Model file for the job. Use its own axes, mm. A direction names the side the tool comes from. Round coordinates to 2 decimals unless told otherwise and drop trailing zeros. Write each loop counter-clockwise with the first axis right and the second up, starting at its lowest first coordinate (ties: lowest second). Pieces come first, ordered by that corner, then holes.
```python
from build123d import *

# Parameters (mm, degrees)
F0_R     = 6.35
F1_DEPTH = 7.62
F2_R     = 3.048
F3_DEPTH = 19.05
F4_R     = 3.048
F5_DEPTH = 19.05


with BuildPart() as f1:
    # F0 (on Front) → F1 (new body)
    with BuildSketch(Plane.XZ):
        Circle(F0_R)
    extrude(amount=F1_DEPTH)

    # F2 (on face) → F3 (join)
    with BuildSketch(Plane(origin=(0, 0, 0), x_dir=(-1, 0, 0), z_dir=(0, 1, 0))):
        Circle(F2_R)
    extrude(amount=F3_DEPTH)

    # F4 (on face) → F5 (join)
    with BuildSketch(Plane.XZ.offset(7.62)):
        Circle(F4_R)
    extrude(amount=F5_DEPTH)


solid = f1.part
```
1) Cut at D-D on z = -3.75. List the corners of the cut face in (x, y), and give its area (3 significant figures).
2) Cut at B-B on x = 0. List the corners of the cut face in (y, z), and give its area (3 significant figures).
3) Cut at A-A on z = 0. List the corners of the cut face in (x, y), and give its area (3 significant figures).
4) Which spindle directions (+Z, -Z, +X, -X, +Y, -Y) get a long thin tool onto all of the face, cutting with end or side? Do faces 3 (the face through (0, -26.67, 0)), 4 (the face through (-0.4, -17.01, 3.02)), 5 (the face through (3, 0, 2)). Say none if no direction does.
5) Flat gauge pins, fed straight in: pin 1 Ø6 at (y, z) = (14.5, 3.5) entering from -X; pin 2 Ø5 at (x, y) = (5, -15) entering from +Z; pin 3 Ø1.5 at (y, z) = (-5.5, -3.5) entering from +X. Where does each tip first touch, or does it go through?
6) Cut at C-C on y = -15.5. List the corners of the cut face in (x, z), and give its area (3 significant figures).
7) Pull direction X, two halves, no side cores. Call faces 1 (the face through (-1.38, -3.76, -6.2)), 2 (the face through (0, 19.05, 0)): released by +X, released by -X, zero draft, split by the parting line, or undercut.
8) Wall check: probe 1 along Y at (x, z) = (-2.75, 5); probe 2 along Z at (x, y) = (-0.25, -20); probe 3 along X at (y, z) = (-1, -5.25). Give the ranges that are in metal, low to high.
Result sheet:
1. outline: (-5.12, -7.62) - (5.12, -7.62) - (5.12, 0) - (-5.12, 0) - close
1. area: 78.1 mm2
2. outline: (-26.67, -3.05) - (-7.62, -3.05) - (-7.62, -6.35) - (0, -6.35) - (0, -3.05) - (19.05, -3.05) - (19.05, 3.05) - (0, 3.05) - (0, 6.35) - (-7.62, 6.35) - (-7.62, 3.05) - (-26.67, 3.05) - close
2. area: 329 mm2
3. outline: (-6.35, -7.62) - (-3.05, -7.62) - (-3.05, -26.67) - (3.05, -26.67) - (3.05, -7.62) - (6.35, -7.62) - (6.35, 0) - (3.05, 0) - (3.05, 19.05) - (-3.05, 19.05) - (-3.05, 0) - (-6.35, 0) - close
3. area: 329 mm2
4. face 3: +Z, -Z, +X, -X, -Y
4. face 4: -Y
4. face 5: +Y
5. pin 1: stops at x = -3.01
5. pin 2: stops at z = 1.74
5. pin 3: stops at x = 5.72
6. outline: circle Ø6.1 at (0, 0)
6. area: 29.2 mm2
7. face 1: split by the parting line
7. face 2: zero draft
8. probe 1: y = -7.62 to 0
8. probe 2: z = -3.04 to 3.04
8. probe 3: x = -3.57 to 3.57
